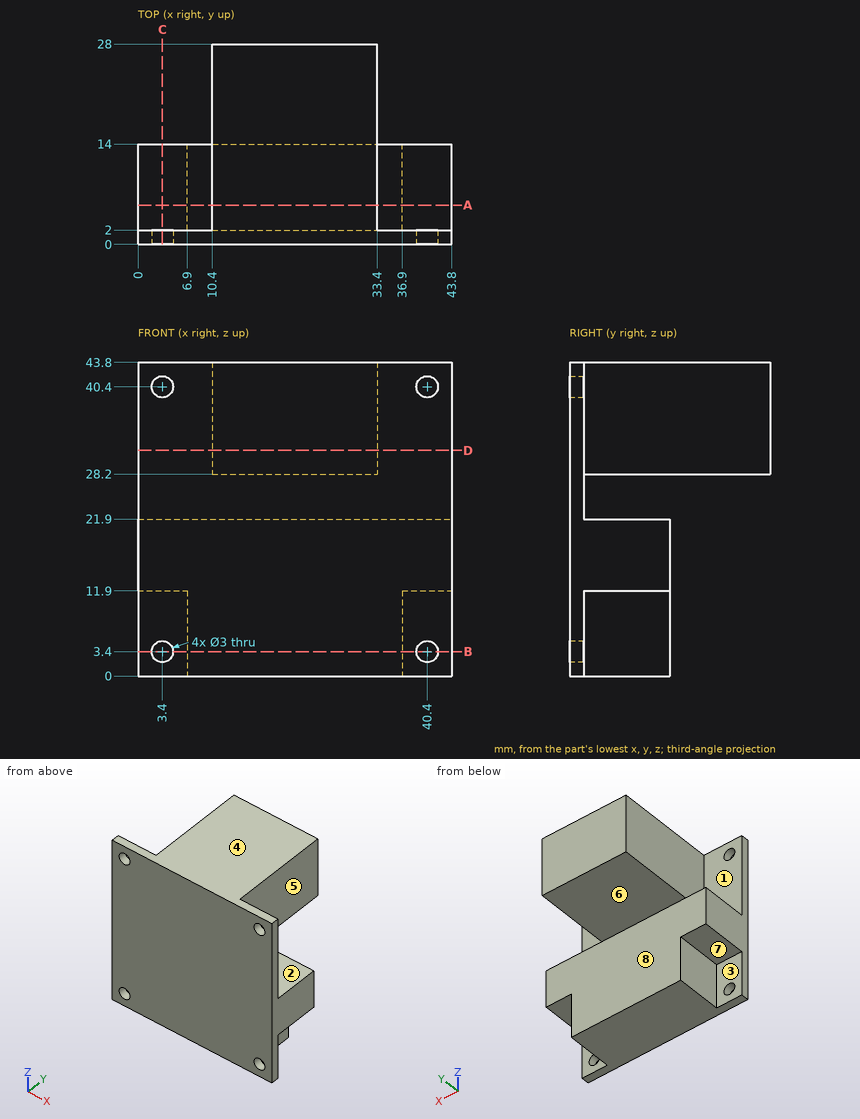
Here's the drawing with two shaded views (mm, measured from the low corner). I have some questions. A direction names the side the tool comes from. Coordinates: 2 decimals unless noted, no trailing zeros. Loops run counter-clockwise (first coordinate to the right, second up) from the corner with the lowest first, then second, coordinate; pieces in that order, holes last. Notation, with made-up numbers: (24.25, 35) -> (45.25, 35) arc R22 cw to (45.25, 66) -> close; hole circle Ø8 at (64, 1.5). An arc over 180 degrees is marked (long way). Answer as a JSON object with one key per item and string values.
1) Thinking about a two-plate mould opening in Z: for the marked faces 1, 2, 3 and 4, which applies, pulls with the +Z half, pulls with the -Z half, needs draft (parallel to the pull), parting line crosses it, or undercut?
Results:
{"face 1": "undercut", "face 2": "undercut", "face 3": "needs draft", "face 4": "pulls with the +Z half"}
2) Imagine slicing it at B-B (z = 3.4). Please give me the cut outline in (x, y).
Results:
{"outline": "(0, 0) -> (1.9, 0) -> (1.9, 2) -> (0, 2) -> close; (4.9, 0) -> (38.9, 0) -> (38.9, 2) -> (36.9, 2) -> (36.9, 14) -> (6.9, 14) -> (6.9, 2) -> (4.9, 2) -> close; (41.9, 0) -> (43.8, 0) -> (43.8, 2) -> (41.9, 2) -> close"}
3) Imagine slicing it at A-A (y = 5.5). Please give me the cut outline in (x, z).
Results:
{"outline": "(0, 11.9) -> (6.9, 11.9) -> (6.9, 0) -> (36.9, 0) -> (36.9, 11.9) -> (43.8, 11.9) -> (43.8, 21.9) -> (0, 21.9) -> close; (10.4, 28.2) -> (33.4, 28.2) -> (33.4, 43.8) -> (10.4, 43.8) -> close"}
4) Imagine slicing it at D-D (z = 31.5). Please give me the cut outline in (x, y).
Results:
{"outline": "(0, 0) -> (43.8, 0) -> (43.8, 2) -> (33.4, 2) -> (33.4, 28) -> (10.4, 28) -> (10.4, 2) -> (0, 2) -> close"}
5) For P1, Ø7.5, axis at x = 2.5, z = 4.5, coming from the +Y side; P2, Ø5.5, axis at x = 4, y = 6, coming from the -Z side; P3, Ø3.5, axis at y = 8, z = 8, coming from the -X side, each with a flat end and sliding along its axis, tell me the tip position at first contact or that it passes through.
Results:
{"P1": "stops at y = 2", "P2": "stops at z = 11.9", "P3": "stops at x = 6.9"}
6) If I drill on line 1 (X direction, y = 1.55, z = 40.4); line 2 (Z direction, x = 26.5, y = 5.75); line 3 (Z direction, x = 4.5, y = 4.75), over which ranges is the centre line in solid material (lowest first)?
Results:
{"line 1": "x = 0 to 1.9, 4.9 to 38.9, 41.9 to 43.8", "line 2": "z = 0 to 21.9, 28.2 to 43.8", "line 3": "z = 11.9 to 21.9"}
7) Imagine slicing it at C-C (x = 3.4). Please give me the cut outline in (y, z).
Results:
{"outline": "(0, 0) -> (2, 0) -> (2, 1.9) -> (0, 1.9) -> close; (0, 4.9) -> (2, 4.9) -> (2, 11.9) -> (14, 11.9) -> (14, 21.9) -> (2, 21.9) -> (2, 38.9) -> (0, 38.9) -> close; (0, 41.9) -> (2, 41.9) -> (2, 43.8) -> (0, 43.8) -> close"}
8) For the marked faces 5, 6, 7 and 8, which set-ups out of +Z, -Z, +X, -X, +Y, -Y let a thin tool reach every point of the face, with its end or its side?
Results:
{"face 5": "+Z, +X, +Y", "face 6": "+X, -X, +Y", "face 7": "-Z, -X, +Y", "face 8": "-Z, +X, -X, +Y"}
